Work out the finished part from the listing and answer in its coordinate system (mm). Face numbers are marked on the shaded views. A direction names the side the tool comes from. Give positions to 0.01 mm unless a question says otherwise; leave off trailing zeros. Order: outer loops, then holes, each group sorted by start corner. A loop starts at its lowest first (then second) coordinate and runs counter-clockwise, first axis right, second up. Notation, with made-up numbers: (-22.75, 18) - (8.25, 18) arc R25 cw to (8.25, 37) - close; hole circle Ø2 at (20.5, -1). An arc over 180 degrees is marked (long way). Put each result on its own line as item: value.
```python
from build123d import *

# Parameters (mm, degrees)
F0_W           = 9
F0_H           = 10
F0_W_2         = 4.3
F0_W_3         = 7.4
F1_DEPTH       = 9
F2_D           = 4
F2_DEPTH       = 12
F2_CBORE_D     = 6.5
F2_CBORE_DEPTH = 3
F2_TIP         = 1.2017212381
F3_DEPTH       = 18
F4_DEPTH       = 28
F5_T1_DEPTH    = 62.5618683077
F6_R           = 2
F7_R           = 0.5


# Not quite as in the source:
# - a fillet or chamfer that OpenCascade refuses, or shapes differently, is made with other operations: its cross-section is extruded or revolved along the edge and cut away or added


with BuildPart() as f1:
    # F0 (on Front) → F1 (new body)
    with BuildSketch(Plane.XZ):
        with Locations((-4.5, 5)):
            Rectangle(F0_W, F0_H)
        with Locations((-11.15, 5)):
            Rectangle(F0_W_2, F0_H)
        with Locations((-17, 5)):
            Rectangle(F0_W_3, F0_H)
        with Locations((-22.85, 5)):
            Rectangle(F0_W_2, F0_H)
        with Locations((-29.5, 5)):
            Rectangle(F0_W, F0_H)
    extrude(amount=F1_DEPTH)

    # F2
    with Locations(Plane(origin=(0, 0, 0), x_dir=(1, 0, 0), z_dir=(0, 1, 0))):
        with Locations((-29.25, -5), (-4.75, -5)):
            CounterBoreHole(F2_D / 2, F2_CBORE_D / 2, F2_CBORE_DEPTH, depth=F2_DEPTH)
            with Locations((0, 0, -(F2_DEPTH + F2_TIP / 2))):  # 118° drill point
                Cone(0, F2_D / 2, F2_TIP, mode=Mode.SUBTRACT)

    # F0 (on Front) → F3 (join)
    with BuildSketch(Plane.XZ):
        with Locations((-22.85, 5)):
            Rectangle(F0_W_2, F0_H)
        with Locations((-17, 5)):
            Rectangle(F0_W_3, F0_H)
        with Locations((-11.15, 5)):
            Rectangle(F0_W_2, F0_H)
    extrude(amount=-F3_DEPTH)

    # F0 (on Front) → F4 (join)
    with BuildSketch(Plane.XZ):
        with Locations((-17, 5)):
            Rectangle(F0_W_3, F0_H)
    extrude(amount=-F4_DEPTH)

    # F5: fillet of radius 15 on 2 edges, made by hand

    # F5_s2 → F5_t1 (cut)
    with BuildSketch(Plane.XY.offset(-26.2809341539)):
        with BuildLine():
            ThreePointArc((-13.3, 18), (-10.1165566231, 13.1665346843), (-9, 7.4876263385))
            Line((-9, 7.4876263385), (-9, 18))
            Line((-9, 18), (-13.3, 18))
        make_face()
        with BuildLine():
            ThreePointArc((-25, 7.4876263385), (-23.8834433769, 13.1665346843), (-20.7, 18))
            Line((-20.7, 18), (-25, 18))
            Line((-25, 18), (-25, 7.4876263385))
        make_face()
    extrude(amount=F5_T1_DEPTH, mode=Mode.SUBTRACT)

    # F6
    f6_edges = [f1.edges().sort_by_distance(p)[0] for p in [
        (0, -4.5, 10),
        (0, -4.5, 0),
        (-34, -4.5, 0),
        (-34, -4.5, 10),
    ]]
    fillet(f6_edges, radius=F6_R)

    # F7
    f7_edges = [f1.edges().sort_by_distance(p)[0] for p in [
        (-9, 0, 5),
        (-25, 0, 5),
        (-25, 7.487626, 5),
        (-20.7, 18, 5),
        (-13.3, 18, 5),
        (-13.3, 28, 5),
        (-20.7, 28, 5),
        (-17, 28, 10),
        (-20.7, 23, 10),
        (-10.116557, 13.166535, 10),
        (-17, -9, 10),
        (0, 0, 5),
        (0, -9, 5),
        (-5.5, 0, 0),
        (-0.585786, 0, 0.585786),
        (-5.5, 0, 10),
        (-0.585786, 0, 9.414214),
        (-0.585786, -9, 0.585786),
        (-0.585786, -9, 9.414214),
        (-17, -9, 0),
        (-33.414214, -9, 0.585786),
        (-33.414214, -9, 9.414214),
        (-34, -9, 5),
        (-28.5, 0, 0),
        (-25, 3.743813, 0),
        (-23.883443, 13.166535, 0),
        (-20.7, 23, 0),
        (-9, 3.743813, 0),
        (-13.3, 23, 0),
        (-10.116557, 13.166535, 0),
        (-9, 3.743813, 10),
        (-13.3, 23, 10),
        (-28.5, 0, 10),
        (-25, 3.743813, 10),
        (-23.883443, 13.166535, 10),
        (-33.414214, 0, 0.585786),
        (-33.414214, 0, 9.414214),
        (-34, 0, 5),
    ]]
    fillet(f7_edges, radius=F7_R)


solid = f1.part
```
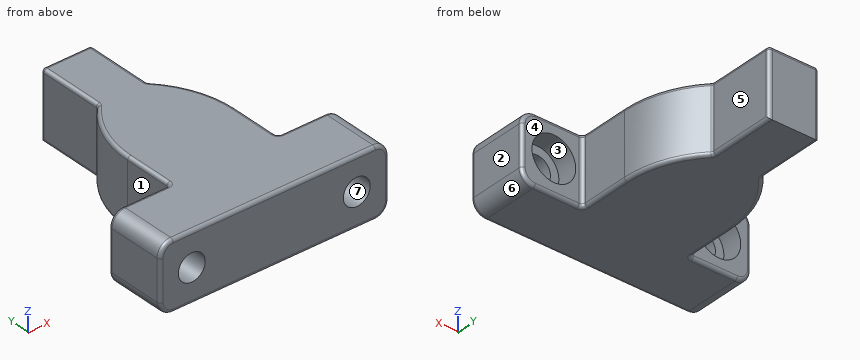
(1) Section D-D, the plane z = 5 is taken. Count the separate pieces of the cut face and the enclosed holes in it, then the cut area to 3 significant figures.
Geometry check:
separate pieces: 3
enclosed holes: 0
area: 553 mm²
(2) Determine the mould class of the marked faces 5, 6 and 7 for opening direction Z: pulls with the +Z half, pulls with the -Z half, needs draft (parallel to the pull), parting line crosses it, or undercut.
Geometry check:
face 5: needs draft
face 6: pulls with the -Z half
face 7: undercut
(3) Straight lines are drawn through the part: line 1 (Z direction, x = -29.25, y = -1.8); line 2 (Y direction, x = -32, z = 4); line 3 (Y direction, x = -26, z = 1.5). For each, find the intervals that lie inside material, in ascending order.
Geometry check:
line 1: z = 0 to 1.75, 8.25 to 10
line 2: y = -9 to -3
line 3: y = -9 to 0
(4) Section B-B, the plane x = -29.25 is taken. Write down the section's boundary in (y, z).
Geometry check:
outline: (-9, 0.5) arc R0.5 ccw to (-8.5, 0) - (-0.5, 0) arc R0.5 ccw to (0, 0.5) - (0, 1.75) - (-3, 1.75) - (-3, 3) - (-9, 3) - close; (-9, 7) - (-3, 7) - (-3, 8.25) - (0, 8.25) - (0, 9.5) arc R0.5 ccw to (-0.5, 10) - (-8.5, 10) arc R0.5 ccw to (-9, 9.5) - close
(5) A tool of negligible diameter and unlimited length cuts with its end or side. For the marked faces 1, 2, 3 and 4, from which of +Z, -Z, +X, -X, +Y, -Y can it reach the whole face along a straight path? Write none if from no direction.
Geometry check:
face 1: +Z, -Z, -X, +Y
face 2: +Z, -Z, +X, +Y, -Y
face 3: +Y
face 4: +Z, -Z, +X, +Y
(6) Section A-A, the plane y = -7 is taken. Write down the section's boundary in (x, z).
Geometry check:
outline: (-34, 2) arc R2 ccw to (-32, 0) - (-2, 0) arc R2 ccw to (0, 2) - (0, 8) arc R2 ccw to (-2, 10) - (-32, 10) arc R2 ccw to (-34, 8) - close; hole circle Ø4 at (-29.25, 5); hole circle Ø4 at (-4.75, 5)
(7) Section C-C, the plane y = 3 is taken. Write down the section's boundary in (x, z).
Geometry check:
outline: (-25, 0.5) arc R0.5 ccw to (-24.5, 0) - (-9.5, 0) arc R0.5 ccw to (-9, 0.5) - (-9, 9.5) arc R0.5 ccw to (-9.5, 10) - (-24.5, 10) arc R0.5 ccw to (-25, 9.5) - close
(8) Given pin 1 (2.5 mm diameter, centred on x = -5.5, z = 6.5, fed in from +Y); pin 2 (1.5 mm diameter, centred on x = -20, y = 24, fed in from -Z); pin 3 (4.5 mm diameter, centred on y = 20.5, z = 3.5, fed in from -X); pin 4 (3 mm diameter, centred on y = 14.5, z = 3.5, fed in from +X), each flat-ended and moving along its own axis, determine where each tip first touches the part or whether it passes through.
Geometry check:
pin 1: stops at y = -3
pin 2: stops at z = 0
pin 3: stops at x = -20.7
pin 4: stops at x = -10.05
